Geometry check sheet. Reference: the model listing, model coordinates, mm. A direction names the side the tool comes from. Round coordinates to 2 decimals unless told otherwise and drop trailing zeros. Write each loop counter-clockwise with the first axis right and the second up, starting at its lowest first coordinate (ties: lowest second). Pieces come first, ordered by that corner, then holes. Notation, with made-up numbers: M 59.25,-38.5 L 118.25,-38.5 A37 ccw 118.25,0.5 Z; hole C 24.5,71.25 d10. An arc over 180 degrees is marked long. One line per item, written item: value. Start each with the question number.
1. Depth check by flat-ended pin: P1, Ø3.5, axis at y = 11, z = 4, coming from the +X side. Enter the tip coordinate at first touch or a pass-through.
2. Section check A-A (x = 16). Record the boundary of the cut face in (y, z), and give its area (3 significant figures).
3. Section check C-C (z = 1). Record the boundary of the cut face in (x, y), and give its area (3 significant figures).
4. Release check for a two-part mould opening along Y. For faces 3 (the flat face through (-2, 0, -0.8)), 4 (the flat face through (120, 1, 3)), 5 (the flat face through (44, 17.5, 3)) record: pulls with the +Y half, pulls with the -Y half, needs draft (parallel to the pull), parting line crosses it, or undercut.
5. Section check B-B (x = 122.5). Record the boundary of the cut face in (y, z).
6. Scan lines: probe 1 along Y at (x, z) = (38, 0.5); probe 2 along Y at (x, z) = (134.5, 3.75); probe 3 along X at (y, z) = (-11.5, 4.75). Record each from-to range of solid material in increasing order. Write a range as [from, to].
7. Access from +Z, -Z, +X, -X, +Y, -Y to the whole of each face (thin tool, end or side, straight path). Record for faces 1 (the flat face through (-2, 0, 6)), 2 (the flat face through (61, 9.555, 3)).
8. Section check D-D (y = 3). Record the boundary of the cut face in (x, z), and give its area (3 significant figures).
from build123d import *

# Parameters (mm, degrees)
F1_DEPTH    = 6
F2_DEPTH    = 0.8
F3_T1_DEPTH = 431.7925725323
F4_DEPTH    = 30


# Not quite as in the source:
# - a fillet or chamfer that OpenCascade refuses, or shapes differently, is made with other operations: its cross-section is extruded or revolved along the edge and cut away or added


with BuildPart() as f1:
    # F0 (on Top) → F1 (new body)
    with BuildSketch(Plane.XY):
        Polygon((150, 17.5), (-150, 17.5), (-150, -17.5), (150, -17.5), (150, -11.1123658717), (0, -11.1123658717), (0, -8.0123320222), (150, -8.0123320222), (150, 9.5545258373), (0, 9.5545258373), (0, 12.9128964618), (150, 12.9128964618), align=None)
    extrude(amount=F1_DEPTH)

    # F2 (add): faces of the model
    f2_faces = [f1.faces().sort_by_distance(p)[0] for p in [
        (-7.6230433236, -0.1272136786, 0),
        (-7.6230433236, -0.1272136786, 6),
    ]]
    extrude(f2_faces, amount=F2_DEPTH, dir=(0, 0, -1))

    # F3: fillet of radius 120.7106781187 on 1 edges, made by hand

    # F3_s2 → F3_t1 (cut)
    with BuildSketch(Plane.XY.offset(-213.2962862662)):
        with BuildLine():
            ThreePointArc((-65.0014854935, 17.5), (-110.9627394699, 8.4075593911), (-150, -17.5))
            Line((-150, -17.5), (-150, 17.5))
            Line((-150, 17.5), (-65.0014854935, 17.5))
        make_face()
    extrude(amount=F3_T1_DEPTH, mode=Mode.SUBTRACT)

    # F4 (cut): a face of the model
    f4_faces = [f1.faces().sort_by_distance(p)[0] for p in [
        (150, 0.7710969076, 2.6),
    ]]
    extrude(f4_faces, amount=-F4_DEPTH, mode=Mode.SUBTRACT)


solid = f1.part
Result sheet:
1. P1: stops at x = 120
2. outline: M -17.5,-0.8 L -11.11,-0.8 L -11.11,6 L -17.5,6 Z; M -8.01,-0.8 L 9.55,-0.8 L 9.55,6 L -8.01,6 Z; M 12.91,-0.8 L 17.5,-0.8 L 17.5,6 L 12.91,6 Z
2. area: 194 mm2
3. outline: M -150,-17.5 L 150,-17.5 L 150,-11.11 L 0,-11.11 L 0,-8.01 L 120,-8.01 L 120,9.55 L 0,9.55 L 0,12.91 L 150,12.91 L 150,17.5 L -65,17.5 A120.71 ccw Z
3. area: 8,080 mm2
4. face 3: needs draft
4. face 4: undercut
4. face 5: pulls with the +Y half
5. outline: M -17.5,-0.8 L -11.11,-0.8 L -11.11,6 L -17.5,6 Z; M 12.91,-0.8 L 17.5,-0.8 L 17.5,6 L 12.91,6 Z
6. probe 1: y = [-17.5, -11.11], [-8.01, 9.55], [12.91, 17.5]
6. probe 2: y = [-17.5, -11.11], [12.91, 17.5]
6. probe 3: x = [-143.49, 150]
7. face 1: +Z, +X, -X, +Y, -Y
7. face 2: +Z, -Z, +X
8. outline: M -122.36,-0.8 L 120,-0.8 L 120,6 L -122.36,6 Z
8. area: 1,650 mm2
